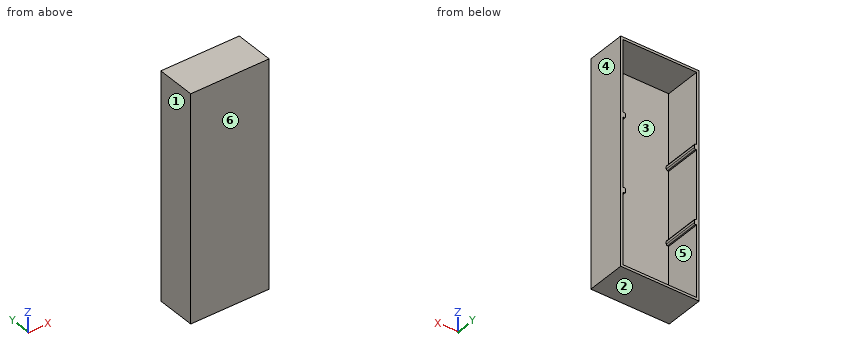
Autodesk Inventor part; units mm, degrees
ref_plane "YZ Plane" through (0, 0, 0) normal (1, 0, 0) x (0, 1, 0)
ref_plane "XZ Plane" through (0, 0, 0) normal (0, 1, 0) x (-1, 0, 0)
ref_plane "XY Plane" through (0, 0, 0) normal (0, 0, 1) x (1, 0, 0)
sketch "Эскиз1" plane through (0, 0, 0) normal (0, 1, 0) x (-1, 0, 0)
  line L0 (0, 0) -> (-300, 0)
  line L1 (-300, 0) -> (-300, -900)
  line L2 (-300, -900) -> (0, -900)
  line L3 (0, -900) -> (0, 0)
  line L4 (-300, 0) -> (0, 0)
  line L5 (0, 0) -> (0, -300)
  line L6 (0, -300) -> (-300, -300)
  line L7 (-300, -300) -> (-300, 0)
  line L8 (0, -900) -> (-300, -900)
  line L9 (-300, -900) -> (-300, -600)
  line L10 (-300, -600) -> (0, -600)
  line L11 (0, -600) -> (0, -900)
  dimension "d0" = 300
  dimension "d1" = 900
extrude "Выдавливание1" add sketch "Эскиз1" along normal blind 10
sketch "Эскиз2" plane through (0, 0, 0) normal (0, -1, 0) x (1, 0, 0)
  line L0 (0, -900) -> (0, 0)
  line L1 (0, 0) -> (-10, 0)
  line L2 (-10, 0) -> (-10, -900)
  line L3 (-10, -900) -> (0, -900)
  line L4 (0, -900) -> (0, 0)
  line L5 (0, 0) -> (300, 0)
  line L6 (300, 0) -> (310, 0)
  line L7 (310, 0) -> (310, -900)
  line L8 (310, -900) -> (300, -900)
  line L9 (300, -900) -> (300, 0)
  line L10 (-10, -900) -> (310, -900)
  line L11 (310, -900) -> (310, -910)
  line L12 (310, -910) -> (-10, -910)
  line L13 (-10, -910) -> (-10, -900)
  line L14 (-10, 0) -> (310, 0)
  line L15 (310, 0) -> (310, 10)
  line L16 (310, 10) -> (-10, 10)
  line L17 (-10, 10) -> (-10, 0)
  dimension "d8" = 10
  dimension "d9" = 10
  dimension "d10" = 10
  dimension "d11" = 10
extrude "Выдавливание2" add sketch "Эскиз2" against normal blind 160 contours L3 L2 L1 L0 | L10 L8 L11 L12 L13 L3 | L1 L17 L16 L15 L6 L5 | L9 L6 L7 L8
ref_plane "РабПлоскость2" through (150, 0, 10) normal (1, 0, 0) x (0, 0, -1)
ref_plane "РабПлоскость3" through (-10, 0, -450) normal (0, 0, 1) x (1, 0, 0)
sketch "Эскиз3" plane through (0, 10, 0) normal (0, 1, 0) x (1, 0, 0)
  line L0 (300, 0) -> (0, 0)
  line L1 (300, 0) -> (300, 300)
  line L2 (300, 900) -> (300, 0)
  line L3 (300, 300) -> (300, 600)
  line L4 (310, -10) -> (310, 910)
  line L5 (290, 610) -> (310, 610)
  line L6 (310, 610) -> (310, 590)
  line L7 (310, 590) -> (290, 590)
  line L8 (290, 590) -> (290, 610)
  line L9 (290, 610) -> (310, 590) construction
  line L10 (310, 610) -> (290, 590) construction
  line L11 (290, 310) -> (310, 310)
  line L12 (310, 310) -> (310, 290)
  line L13 (310, 290) -> (290, 290)
  line L14 (290, 290) -> (290, 310)
  line L15 (290, 310) -> (310, 290) construction
  line L16 (310, 310) -> (290, 290) construction
  line L17 (10, 610) -> (-10, 610)
  line L18 (-10, 610) -> (-10, 590)
  line L19 (-10, 590) -> (10, 590)
  line L20 (10, 590) -> (10, 610)
  line L21 (0, 0) -> (0, 900)
  line L22 (10, 610) -> (-10, 590) construction
  line L23 (-10, 610) -> (10, 590) construction
  line L24 (-10, 910) -> (-10, -10)
  line L25 (10, 310) -> (-10, 310)
  line L26 (-10, 310) -> (-10, 290)
  line L27 (-10, 290) -> (10, 290)
  line L28 (10, 290) -> (10, 310)
  line L29 (10, 310) -> (-10, 290) construction
  line L30 (-10, 310) -> (10, 290) construction
  point P0 (0, 600)
  point P1 (0, 300)
  point P2 (0, 310)
  point P3 (0, 590)
  point P4 (300, 590)
  point P5 (300, 310)
  dimension "d14" = 300
  dimension "d15" = 300
  dimension "d16" = 20
  dimension "d17" = 20
extrude "Выдавливание3" add sketch "Эскиз3" along normal blind 150
fillet "Сопряжение1" radius 5 8 edges at (290, 85, -610) (290, 85, -590) (290, 85, -310) (290, 85, -290) (10, 85, -310) (10, 85, -290) (10, 85, -610) (10, 85, -590)
properties part number "lab"
Can you work these out from the model? Positions are in its coordinate system, mm. Face numbers are marked on the shaded views. A direction names the side the tool comes from. Round coordinates to 2 decimals unless told otherwise and drop trailing zeros. Loops run counter-clockwise (first coordinate to the right, second up) from the corner with the lowest first, then second, coordinate; pieces in that order, holes last. Notation, with made-up numbers: (44, 45) -> (72, 45) arc R21 ccw to (72, 64) -> close; hole circle Ø10 at (56, 84). An arc over 180 degrees is marked (long way). Answer in a Markdown table with one row per item.
Item 1: If I drill on probe 1 along X at (y, z) = (65.5, -342); probe 2 along Z at (x, y) = (8.5, 118.5); probe 3 along Z at (x, y) = (258, 60), over which ranges is the centre line in solid material (lowest first)?
Answer block:
| item | result |
|---|---|
| probe 1 | -10 to 0, 300 to 310 |
| probe 2 | -910 to -900, -608.57 to -591.43, -308.57 to -291.43, 0 to 10 |
| probe 3 | -910 to -900, 0 to 10 |
Item 2: We'd pull the mould along X, two halves only. Please class the marked faces 1, 2, 3 and 4: released by +X, released by -X, zero draft, split by the parting line, or undercut.
Answer block:
| item | result |
|---|---|
| face 1 | released by -X |
| face 2 | zero draft |
| face 3 | undercut |
| face 4 | released by +X |
Item 3: On a 3-axis mill with a long thin cutter (end or side, diameter ignored), from which of +Z, -Z, +X, -X, +Y, -Y can I reach the whole of each face in a straight line? I mean the marked faces 5 and 6. Say none if no direction works.
Answer block:
| item | result |
|---|---|
| face 5 | +Y |
| face 6 | +Z, -Z, +X, -X, -Y |
Item 4: Suppose I cut it at C-C, the plane z = -800. List the corners of the cut face in (x, y) for me.
Answer block:
| item | result |
|---|---|
| outline | (-10, 0) -> (310, 0) -> (310, 160) -> (300, 160) -> (300, 10) -> (0, 10) -> (0, 160) -> (-10, 160) -> close |
Item 5: Suppose I cut it at B-B, the plane x = 21. List the corners of the cut face in (y, z) for me.
Answer block:
| item | result |
|---|---|
| outline | (0, -910) -> (160, -910) -> (160, -900) -> (10, -900) -> (10, 0) -> (160, 0) -> (160, 10) -> (0, 10) -> close |
